```python
from build123d import *

# Parameters (mm, degrees)
SKETCH_1_R               = 2.05
EXTRUDE_1_DEPTH          = 3
PATTERN_CIRCULAR_1_COUNT = 7
PATTERN_CIRCULAR_1_ANGLE = 162
CHAMFER_1_SIZE           = 0.5
CHAMFER_2_SIZE           = 0.5
CHAMFER_3_SIZE           = 0.3
EXTRUDE_2_DEPTH          = 3


with BuildPart() as part:
    # 스케치1 → 보스-돌출1 (new, symmetric)
    with BuildSketch(Plane.XY):
        with BuildLine():
            ThreePointArc((-0.75, 4.183300133), (0, -4.25), (0.75, 4.183300133))
            Line((0.75, 4.183300133), (0.621752267, 4.811019676))
            Line((0.621752267, 4.811019676), (0.4, 5.284884105))
            ThreePointArc((0.4, 5.284884105), (0, 5.3), (-0.4, 5.284884105))
            Line((-0.4, 5.284884105), (-0.621752267, 4.811019676))
            Line((-0.621752267, 4.811019676), (-0.75, 4.183300133))
        make_face()
        Circle(SKETCH_1_R, mode=Mode.SUBTRACT)
    extrude_1 = extrude(amount=EXTRUDE_1_DEPTH, both=True)

    # 원형 패턴1: 보스-돌출1 ×7 about axis
    pattern_circular_1_axis = Axis((0, 0, 0), (0, 0, -1))
    for i in range(1, PATTERN_CIRCULAR_1_COUNT):
        add(extrude_1.rotate(pattern_circular_1_axis, i * PATTERN_CIRCULAR_1_ANGLE / (PATTERN_CIRCULAR_1_COUNT - 1)))

    # 모따기1
    chamfer_1_edges = [part.edges().sort_by_distance(p)[0] for p in [
        (0, 5.3, -3),
        (1.63779007, -5.040599536, -3),
        (3.74766594, -3.74766594, -3),
        (5.040599536, -1.63779007, -3),
        (5.234748205, 0.829102665, -3),
        (4.28779007, 3.115261837, -3),
        (2.406149649, 4.722334578, -3),
    ]]
    chamfer(chamfer_1_edges, length=CHAMFER_1_SIZE)

    # 모따기2
    chamfer_2_edges = [part.edges().sort_by_distance(p)[0] for p in [
        (0, 5.3, 3),
        (2.406149649, 4.722334578, 3),
        (4.28779007, 3.115261837, 3),
        (5.234748205, 0.829102665, 3),
        (5.040599536, -1.63779007, 3),
        (3.74766594, -3.74766594, 3),
        (1.63779007, -5.040599536, 3),
    ]]
    chamfer(chamfer_2_edges, length=CHAMFER_2_SIZE)

    # 모따기3
    chamfer_3_edges = [part.edges().sort_by_distance(p)[0] for p in [
        (-2.05, 0, 3),
        (-2.05, 0, -3),
    ]]
    chamfer(chamfer_3_edges, length=CHAMFER_3_SIZE)

    # 스케치4 → 보스-돌출2 (add, symmetric)
    with BuildSketch(Plane.XY):
        Polygon((-1.055150369, -9.645655488), (0.510208527, -4.219263829), (-3.994308358, -1.451895569), (-3.497178156, -9.809555456), align=None)
    extrude(amount=EXTRUDE_2_DEPTH, both=True)


solid = part.part
```
Input: part model. Units: mm. Frame: model coordinates. Coordinates: 2 decimals unless noted, no trailing zeros. Write each loop counter-clockwise with the first axis right and the second up, starting at its lowest first coordinate (ties: lowest second). Pieces come first, ordered by that corner, then holes.
1) Pin query (flat end, axial travel): pin 1 Ø1.5 at (x, z) = (4, -0.5) entering from -Y; pin 2 Ø4.5 at (x, y) = (0, 0) entering from -Z; pin 3 Ø2 at (x, y) = (1.5, 0) entering from -Z. Return the tip coordinate at first contact, or that it passes through.
2) Material intervals for line 1 along X through (y, z) = (-4.5, 1.75); line 2 along Y through (x, z) = (-1.5, -1); line 3 along Y through (x, z) = (1.5, 1.75), sorted ascending.
3) Section A-A on x = 0. Output: boundary loops of the cut face in (y, z).
4) Mould query, pull axis X, two halves, no side actions, for faces 1 (the cylindrical face through (-0.267, 2.033, -0.038)), 2 (the cylindrical face through (-3.657, 2.165, 0.042)), 3 (the flat face through (-0.8, -2.4, 3)). Classes: pulls with the +X half, pulls with the -X half, needs draft (parallel to the pull), parting line crosses it, or undercut.
Check result:
1. pin 1: stops at y = -4.02
1. pin 2: stops at z = -2.9
1. pin 3: stops at z = -3
2. line 1: x = -3.81 to 0.43, 0.74 to 2.06
2. line 2: y = -9.68 to -1.4, 1.4 to 3.98
2. line 3: y = -5.08 to -1.4, 1.4 to 4.41
3. outline: (-5.99, -3) - (-2.35, -3) - (-2.05, -2.7) - (-2.05, 2.7) - (-2.35, 3) - (-5.99, 3) - close; (2.05, -2.7) - (2.35, -3) - (4.8, -3) - (5.3, -2.5) - (5.3, 2.5) - (4.8, 3) - (2.35, 3) - (2.05, 2.7) - close
4. face 1: undercut
4. face 2: pulls with the -X half
4. face 3: needs draft
